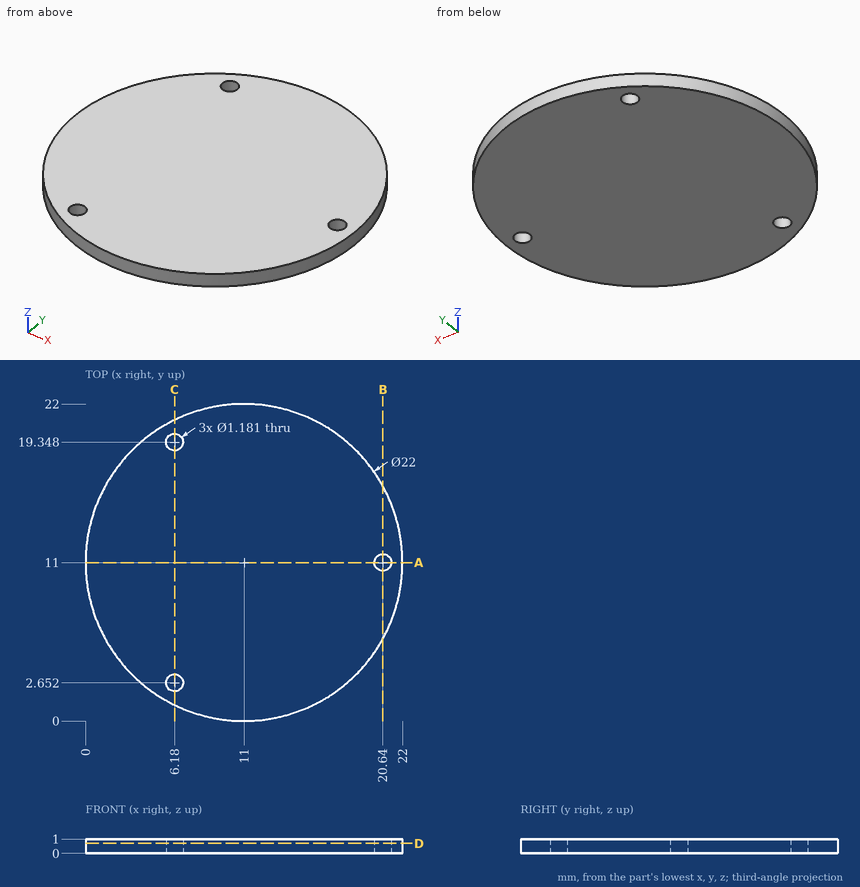
Job drawing, mm, ordinate dimensions from the low corner. One solid piece. Give positions to 0.01 mm unless a question says otherwise; leave off trailing zeros. Loops run counter-clockwise (first coordinate to the right, second up) from the corner with the lowest first, then second, coordinate; pieces in that order, holes last. Notation, with made-up numbers: M 32,46.5 L 44,46.5 A9 ccw 44,62.5 Z; hole C 85.25,-14 d7. An arc over 180 degrees is marked long. Answer in a Markdown table with one row per item. Add a question column.
Item 1: Band-saw the part on C-C on x = 6.18. Give the cut face in (y, z).
Item 2: Band-saw the part on A-A on y = 11. Give the cut face in (x, z).
Item 3: Band-saw the part on B-B on x = 20.64. Give the cut face in (y, z).
Item 4: Probe probe 1 along Y at (x, z) = (11, 0.5); probe 2 along Y at (x, z) = (21, 0.6) (1 decimal); probe 3 along Y at (x, z) = (20.64, 0.65) (1 decimal). List the from-to ranges inside material, lowest first.
Item 5: Band-saw the part on D-D on z = 0.7. Give the cut face in (x, y), then the cut area to 3 significant figures.
Reply:
| question | item | result |
|---|---|---|
| 1 | outline | M 1.11,0 L 2.06,0 L 2.06,1 L 1.11,1 Z; M 3.24,0 L 18.76,0 L 18.76,1 L 3.24,1 Z; M 19.94,0 L 20.89,0 L 20.89,1 L 19.94,1 Z |
| 2 | outline | M 0,0 L 20.05,0 L 20.05,1 L 0,1 Z; M 21.23,0 L 22,0 L 22,1 L 21.23,1 Z |
| 3 | outline | M 5.7,0 L 10.41,0 L 10.41,1 L 5.7,1 Z; M 11.59,0 L 16.3,0 L 16.3,1 L 11.59,1 Z |
| 4 | probe 1 | y = 0 to 22 |
| 4 | probe 2 | y = 6.4 to 10.5, 11.5 to 15.6 |
| 4 | probe 3 | y = 5.7 to 10.4, 11.6 to 16.3 |
| 5 | outline | C 11,11 d22; hole C 6.18,2.65 d1.18; hole C 6.18,19.35 d1.18; hole C 20.64,11 d1.18 |
| 5 | area | 377 mm^2 |
